from build123d import *

# Parameters (mm, degrees)
SKETCH1_R           = 27.94
BOSS_EXTRUDE1_DEPTH = 5
CUT_EXTRUDE2_DEPTH  = 5
SKETCH9_R           = 1.5
SKETCH10_R          = 9
BOSS_EXTRUDE2_DEPTH = 4
CUT_EXTRUDE4_DEPTH  = 4
SKETCH12_R          = 2.5
CUT_EXTRUDE5_DEPTH  = 6


with BuildPart() as part:
    # Sketch1 → Boss-Extrude1 (new body)
    with BuildSketch(Plane.XY):
        Circle(SKETCH1_R)
    extrude(amount=-BOSS_EXTRUDE1_DEPTH)

    # Sketch7 → Cut-Extrude2 (cut)
    with BuildSketch(Plane.XY):
        with BuildLine():
            ThreePointArc((2.122364529, -9.772183421), (1.630852156, -9.866119868), (1.135255991, -9.935350715))
            Line((1.135255991, -9.935350715), (16.158618381, -19.597424627))
            ThreePointArc((16.158618381, -19.597424627), (21.837418082, -12.972554549), (24.939104938, -4.816746297))
            Line((24.939104938, -4.816746297), (2.122364529, -9.772183421))
        make_face()
        with BuildLine():
            Line((14.228656248, -21.040564188), (-5.409238814, -8.410715514))
            ThreePointArc((-5.409238814, -8.410715514), (-5.823213644, -8.129586881), (-6.222606654, -7.828101074))
            Line((-6.222606654, -7.828101074), (-2.431603216, -25.283340479))
            ThreePointArc((-2.431603216, -25.283340479), (6.268405118, -24.6143677), (14.228656248, -21.040564188))
        make_face()
        with BuildLine():
            ThreePointArc((8.410715514, -5.409238814), (8.129586881, -5.823213644), (7.828101074, -6.222606654))
            Line((7.828101074, -6.222606654), (25.283340479, -2.431603216))
            ThreePointArc((25.283340479, -2.431603216), (24.6143677, 6.268405118), (21.040564188, 14.228656248))
            Line((21.040564188, 14.228656248), (8.410715514, -5.409238814))
        make_face()
        with BuildLine():
            Line((-4.816746297, -24.939104938), (-9.772183421, -2.122364529))
            ThreePointArc((-9.772183421, -2.122364529), (-9.866119868, -1.630852156), (-9.935350715, -1.135255991))
            Line((-9.935350715, -1.135255991), (-19.597424627, -16.158618381))
            ThreePointArc((-19.597424627, -16.158618381), (-12.972554549, -21.837418082), (-4.816746297, -24.939104938))
        make_face()
        with BuildLine():
            Line((-21.040564188, -14.228656248), (-8.410715514, 5.409238814))
            ThreePointArc((-8.410715514, 5.409238814), (-8.129586881, 5.823213644), (-7.828101074, 6.222606654))
            Line((-7.828101074, 6.222606654), (-25.283340479, 2.431603216))
            ThreePointArc((-25.283340479, 2.431603216), (-24.6143677, -6.268405118), (-21.040564188, -14.228656248))
        make_face()
        with BuildLine():
            Line((9.935350715, 1.135255991), (19.597424627, 16.158618381))
            ThreePointArc((19.597424627, 16.158618381), (12.972554549, 21.837418082), (4.816746297, 24.939104938))
            Line((4.816746297, 24.939104938), (9.772183421, 2.122364529))
            ThreePointArc((9.772183421, 2.122364529), (9.866119868, 1.630852156), (9.935350715, 1.135255991))
        make_face()
        with BuildLine():
            Line((-24.939104938, 4.816746297), (-2.122364529, 9.772183421))
            ThreePointArc((-2.122364529, 9.772183421), (-1.630852156, 9.866119868), (-1.135255991, 9.935350715))
            Line((-1.135255991, 9.935350715), (-16.158618381, 19.597424627))
            ThreePointArc((-16.158618381, 19.597424627), (-21.837418082, 12.972554549), (-24.939104938, 4.816746297))
        make_face()
        with BuildLine():
            Line((6.222606654, 7.828101074), (2.431603216, 25.283340479))
            ThreePointArc((2.431603216, 25.283340479), (-6.268405118, 24.6143677), (-14.228656248, 21.040564188))
            Line((-14.228656248, 21.040564188), (5.409238814, 8.410715514))
            ThreePointArc((5.409238814, 8.410715514), (5.823213644, 8.129586881), (6.222606654, 7.828101074))
        make_face()
    extrude(amount=-CUT_EXTRUDE2_DEPTH, mode=Mode.SUBTRACT)

    # Sketch9 → Cut-Revolve3 (revolve, cut)
    with BuildSketch(Plane(origin=(0, 0, 0), x_dir=(1, 0, 0), z_dir=(0, 1, 0))):
        with Locations((-27.94, 2.5)):
            Circle(SKETCH9_R)
    revolve(axis=Axis((0, 0, -92.148103423), (0, 0, 1)), mode=Mode.SUBTRACT)

    # Sketch10 → Boss-Extrude2 (add)
    with BuildSketch(Plane(origin=(0, 0, -5), x_dir=(-1, 0, 0), z_dir=(0, 0, -1))):
        Circle(SKETCH10_R)
    extrude(amount=BOSS_EXTRUDE2_DEPTH)

    # Sketch11 → Cut-Extrude4 (cut)
    with BuildSketch(Plane(origin=(0, 0, -9), x_dir=(-1, 0, 0), z_dir=(0, 0, -1))):
        Polygon((7, 0), (3.5, 6.062177826), (-3.5, 6.062177826), (-7, 0), (-3.5, -6.062177826), (3.5, -6.062177826), align=None)
    extrude(amount=-CUT_EXTRUDE4_DEPTH, mode=Mode.SUBTRACT)

    # Sketch12 → Cut-Extrude5 (cut, through all)
    with BuildSketch(Plane(origin=(0, 0, -5), x_dir=(-1, 0, 0), z_dir=(0, 0, -1))):
        Circle(SKETCH12_R)
    extrude(amount=-CUT_EXTRUDE5_DEPTH, mode=Mode.SUBTRACT)


solid = part.part
Build history of the part. All positions in model axes, mm. A direction names the side the tool comes from. Round coordinates to 2 decimals unless told otherwise and drop trailing zeros. Write each loop counter-clockwise with the first axis right and the second up, starting at its lowest first coordinate (ties: lowest second). Pieces come first, ordered by that corner, then holes. Notation, with made-up numbers: M 84.25,26 L 122.25,26 A27 cw 122.25,46 Z; hole C -21,-32 d4. An arc over 180 degrees is marked long. Use CSV: the item, a comma, the result in double quotes.
1. Saw through at C-C (y = -18). State how many separate pieces and enclosed holes the cut face has, plus the area to 3 significant figures.
Reply:
separate pieces,"4"
enclosed holes,"0"
area,"57.5 mm²"
2. Tool access for faces 1 (the face through (-16.434, 4.354, -2.465)), 2 (the face through (6, 0, 0)), 3 (the face through (5.274, -2.989, -7.028)): list every direction of +Z, -Z, +X, -X, +Y, -Y with a clear straight run to the whole face (end or side of a thin tool).
Reply:
face 1,"+Z, -Z"
face 2,"+Z, +X, -X, +Y, -Y"
face 3,"-Z"
3. Saw through at A-A (x = 0). Give the cut face in (y, z).
Reply:
outline,"M -27.94,-5 L -25.4,-5 L -25.4,0 L -27.94,0 L -27.94,-1 A1.5 cw -27.94,-4 Z; M -11.89,-5 L -9,-5 L -9,-9 L -6.06,-9 L -6.06,-5 L -2.5,-5 L -2.5,0 L -11.89,0 Z; M 2.5,-5 L 6.06,-5 L 6.06,-9 L 9,-9 L 9,-5 L 11.89,-5 L 11.89,0 L 2.5,0 Z; M 25.4,-5 L 27.94,-5 L 27.94,-4 A1.5 cw 27.94,-1 L 27.94,0 L 25.4,0 Z"
4. Flat gauge pins, fed straight in: pin 1 (5 mm diameter, centred on x = 3, z = -5, fed in from +Y); pin 2 (12 mm diameter, centred on x = -9.5, y = -22, fed in from -Z); pin 3 (2 mm diameter, centred on x = -1, z = -7, fed in from -Y). Where does each tip first touch, or does it go through?
Reply:
pin 1,"stops at y = 27.94"
pin 2,"stops at z = -5"
pin 3,"stops at y = -9"
5. Two-plate mould, pull along X, no slides. Class faces 4 (the face through (6.1, 2.1, -9)), 5 (the face through (1.172, 8.923, -6.972)), 6 (the face through (24.644, 6.149, -2.465)): +X half, -X half, draft (parallel to the pull), parting line (faces both ways), or undercut.
Reply:
face 4,"draft"
face 5,"parting line"
face 6,"undercut"
6. Saw through at B-B (z = -6.25). Give the cut face in (x, y), plus the area to 3 significant figures.
Reply:
outline,"C 0,0 d18; hole M -7,0 L -3.5,-6.06 L 3.5,-6.06 L 7,0 L 3.5,6.06 L -3.5,6.06 Z"
area,"127 mm²"
7. Wall check: probe 1 along X at (y, z) = (19, -2.25); probe 2 along Y at (x, z) = (22, -3.25); probe 3 along Y at (x, z) = (-0.5, -2.5). Give the ranges that are in metal, low to high. Write a range as from..to.
Reply:
probe 1,"x = -18.42..-16.86, -15.23..-11.06, 3.8..6.11, 16.86..18.42"
probe 2,"y = -15.02..-12.69, -5.46..-3.14, 12.69..15.02"
probe 3,"y = -26.44..-25.4, -11.57..-2.45, 2.45..12.21, 25.4..26.44"
